Model file for the job. Use its own axes, mm. Round coordinates to 2 decimals unless told otherwise and drop trailing zeros. Order: outer loops, then holes, each group sorted by start corner. A loop starts at its lowest first (then second) coordinate and runs counter-clockwise, first axis right, second up. Notation, with made-up numbers: (9.25, 39.5) - (20.25, 39.5) arc R25 cw to (20.25, 76.5) - close; hole circle Ø1 at (-6.75, -3). An arc over 180 degrees is marked (long way). Put each result on its own line as item: value. Start each with the question number.
Item 1: Probe probe 1 along Z at (x, y) = (13.5, 3); probe 2 along Y at (x, z) = (36, 18). List the from-to ranges inside material, lowest first.
Item 2: Saw through at C-C on x = -21.5. List the corners of the cut face in (y, z).
Item 3: Saw through at A-A on y = 17.75. List the corners of the cut face in (x, z), plus the area to 3 significant figures.
Item 4: Pin check, flat tips, straight feed: pin 1 Ø10 at (x, y) = (-15.5, 17) entering from +Z; pin 2 Ø8 at (x, y) = (-10, 10.5) entering from +Z; pin 3 Ø4 at (y, z) = (4.5, -1) entering from +X; pin 4 Ø5 at (x, y) = (16.5, 7.5) entering from -Z. Stop position of each tip, or through.
Item 5: Saw through at B-B on z = -21.5. List the corners of the cut face in (x, y), plus the area to 3 significant figures.
```python
from build123d import *

# Parameters (mm, degrees)
SKETCH_1_W             = 100
SKETCH_1_H             = 100
EXTRUDE_1_DEPTH        = 1.5
SKETCH_2_R             = 0.75
EXTRUDE_2_DEPTH        = 0.75
SKETCH_3_W             = 1.5
SKETCH_3_H             = 3
EXTRUDE_3_DEPTH        = 1.5
SKETCH_5_W             = 3
SKETCH_5_H             = 1.5
EXTRUDE_4_DEPTH        = 3
SKETCH_7_R             = 0.75
EXTRUDE_5_DEPTH        = 2.5
SKETCH_8_W             = 6
SKETCH_8_H             = 9
EXTRUDE_6_DEPTH        = 10.4
SKETCH_9_W             = 3
SKETCH_9_H             = 1.5
EXTRUDE_7_DEPTH        = 4
SKETCH_10_R            = 0.75
EXTRUDE_8_DEPTH        = 3
SKETCH_11_W            = 6
SKETCH_11_H            = 2
CUT_EXTRUDE_1_DEPTH    = 10.4
SKETCH_12_W            = 6
SKETCH_12_H            = 3.5
EXTRUDE_9_DEPTH        = 20.17
SKETCH_13_W            = 3
SKETCH_13_H            = 1.5
EXTRUDE_10_DEPTH       = 4
SKETCH_14_R            = 0.75
EXTRUDE_11_DEPTH       = 2
PATTERN_LINEAR_2_COUNT = 2
PATTERN_LINEAR_2_PITCH = 13.6
SKETCH_16_W            = 6
SKETCH_16_H            = 8.75
CUT_EXTRUDE_2_DEPTH    = 9.25
SKETCH_17_W            = 6
SKETCH_17_H            = 2
CUT_EXTRUDE_3_DEPTH    = 1.65
SKETCH_18_W            = 3
SKETCH_18_H            = 1.5
EXTRUDE_12_DEPTH       = 4
SKETCH_19_R            = 0.75
EXTRUDE_13_DEPTH       = 3
EXTRUDE_14_DEPTH       = 1.5
SKETCH_21_W            = 0.75
SKETCH_21_H            = 3
CUT_EXTRUDE_4_DEPTH    = 1.5
SKETCH_22_W            = 1.5
SKETCH_22_H            = 0.5
EXTRUDE_15_DEPTH       = 2.5
SKETCH_23_W            = 3.5
SKETCH_23_H            = 14.4
CUT_EXTRUDE_5_DEPTH    = 6


with BuildPart() as part:
    # Sketch 1 → Extrude 1 (new body)
    with BuildSketch(Plane(origin=(0, 0, 0), x_dir=(1, 0, 0), z_dir=(0, 1, 0))):
        Rectangle(SKETCH_1_W, SKETCH_1_H)
    extrude(amount=EXTRUDE_1_DEPTH)



with BuildPart() as body_2:
    # Sketch 2 → Extrude 2 (new, symmetric)
    with BuildSketch(Plane.XY):
        with Locations((-40.336831864, 4.5)):
            Circle(SKETCH_2_R)
    extrude(amount=EXTRUDE_2_DEPTH, both=True)


with BuildPart() as part_1:
    add(part.part)

    add(body_2.part)  # Extrude 3 merges body 2
    # Sketch 3 → Extrude 3 (add)
    with BuildSketch(Plane.XY.offset(0.75)):
        with Locations((-40.336831864, 3)):
            Rectangle(SKETCH_3_W, SKETCH_3_H)
    extrude_3 = extrude(amount=EXTRUDE_3_DEPTH)

    # Mirror 1: Extrude 3 across plane
    add(extrude_3.mirror(Plane.XY))

    # Sketch 5 → Extrude 4 (add)
    with BuildSketch(Plane(origin=(0, 4.5, 0), x_dir=(1, 0, 0), z_dir=(0, 1, 0))):
        with Locations((-34.136831864, -0.5)):
            Rectangle(SKETCH_5_W, SKETCH_5_H)
        with Locations((-34.136831864, 3)):
            Rectangle(SKETCH_5_W, SKETCH_5_H)
    extrude(amount=-EXTRUDE_4_DEPTH)

    # Sketch 7 → Extrude 5 (add)
    with BuildSketch(Plane.XY.offset(-2.25)):
        with Locations(Location((-34.136831864, 4.5, 0), (0, 0, 180))):
            Circle(SKETCH_7_R)
    extrude(amount=EXTRUDE_5_DEPTH)

    # Sketch 8 → Extrude 6 (add)
    with BuildSketch(Plane(origin=(0, 1.5, 0), x_dir=(1, 0, 0), z_dir=(0, 1, 0))):
        with Locations((-17.336831864, 1.25)):
            Rectangle(SKETCH_8_W, SKETCH_8_H)
    extrude_6 = extrude(amount=EXTRUDE_6_DEPTH)

    # Sketch 9 → Extrude 7 (add)
    with BuildSketch(Plane(origin=(0, 11.9, 0), x_dir=(1, 0, 0), z_dir=(0, 1, 0))):
        with Locations((-17.336831864, 3)):
            Rectangle(SKETCH_9_W, SKETCH_9_H)
        with Locations((-17.336831864, -0.5)):
            Rectangle(SKETCH_9_W, SKETCH_9_H)
    extrude(amount=EXTRUDE_7_DEPTH)

    # Sketch 10 → Extrude 8 (add)
    with BuildSketch(Plane.XY.offset(-2.25)):
        with Locations(Location((-17.336831864, 14.9, 0), (0, 0, 180))):
            Circle(SKETCH_10_R)
    extrude(amount=EXTRUDE_8_DEPTH)

    # Sketch 11 → Cut-Extrude 1 (cut)
    with BuildSketch(Plane(origin=(0, 11.9, 0), x_dir=(1, 0, 0), z_dir=(0, 1, 0))):
        with Locations((-17.336831864, 1.25)):
            Rectangle(SKETCH_11_W, SKETCH_11_H)
    extrude(amount=-CUT_EXTRUDE_1_DEPTH, mode=Mode.SUBTRACT)

    # Sketch 12 → Extrude 9 (add)
    with BuildSketch(Plane(origin=(0, 1.5, 0), x_dir=(1, 0, 0), z_dir=(0, 1, 0))):
        with Locations((16.243168136, 0)):
            Rectangle(SKETCH_12_W, SKETCH_12_H)
        with Locations((16.243168136, 5.5)):
            Rectangle(SKETCH_12_W, SKETCH_12_H)
    extrude(amount=EXTRUDE_9_DEPTH)

    # Sketch 13 → Extrude 10 (add)
    with BuildSketch(Plane(origin=(0, 21.67, 0), x_dir=(1, 0, 0), z_dir=(0, 1, 0))):
        with Locations((16.243168136, 1)):
            Rectangle(SKETCH_13_W, SKETCH_13_H)
        with Locations((16.243168136, 4.5)):
            Rectangle(SKETCH_13_W, SKETCH_13_H)
    extrude(amount=EXTRUDE_10_DEPTH)

    # Sketch 14 → Extrude 11 (add)
    with BuildSketch(Plane.XY.offset(-3.75)):
        with Locations(Location((16.243168136, 24.67, 0), (0, 0, 180))):
            Circle(SKETCH_14_R)
    extrude(amount=EXTRUDE_11_DEPTH)

    # Pattern Linear 2: Extrude 6 ×2
    with Locations(*[(i * PATTERN_LINEAR_2_PITCH, 0, 0) for i in range(1, PATTERN_LINEAR_2_COUNT)]):
        add(extrude_6)

    # Sketch 16 → Cut-Extrude 2 (cut, symmetric)
    with BuildSketch(Plane.XY):
        with Locations((-3.736831864, 7.525)):
            Rectangle(SKETCH_16_W, SKETCH_16_H)
    extrude(amount=CUT_EXTRUDE_2_DEPTH, both=True, mode=Mode.SUBTRACT)

    # Sketch 17 → Cut-Extrude 3 (cut)
    with BuildSketch(Plane(origin=(0, 3.15, 0), x_dir=(1, 0, 0), z_dir=(0, 1, 0))):
        with Locations((-3.736831864, 1.25)):
            Rectangle(SKETCH_17_W, SKETCH_17_H)
    extrude(amount=-CUT_EXTRUDE_3_DEPTH, mode=Mode.SUBTRACT)

    # Sketch 18 → Extrude 12 (add)
    with BuildSketch(Plane(origin=(0, 3.15, 0), x_dir=(1, 0, 0), z_dir=(0, 1, 0))):
        with Locations((-3.736831864, 3)):
            Rectangle(SKETCH_18_W, SKETCH_18_H)
        with Locations((-3.736831864, -0.5)):
            Rectangle(SKETCH_18_W, SKETCH_18_H)
    extrude(amount=EXTRUDE_12_DEPTH)

    # Sketch 19 → Extrude 13 (add)
    with BuildSketch(Plane.XY.offset(-2.25)):
        with Locations(Location((-3.736831864, 6.15, 0), (0, 0, 180))):
            Circle(SKETCH_19_R)
    extrude(amount=EXTRUDE_13_DEPTH)

    # Sketch 20 → Extrude 14 (add)
    with BuildSketch(Plane(origin=(0, 4.5, 0), x_dir=(1, 0, 0), z_dir=(0, 1, 0))):
        Polygon((-32.636831864, 0.25), (-33.386831864, 0.25), (-33.386831864, -0.25), (-34.886831864, -0.25), (-34.886831864, 0.25), (-35.636831864, 0.25), (-35.636831864, -1.25), (-32.636831864, -1.25), align=None)
        Polygon((-35.636831864, 3.75), (-35.636831864, 2.25), (-34.886831864, 2.25), (-33.386831864, 2.25), (-32.636831864, 2.25), (-32.636831864, 3.75), align=None)
    extrude(amount=EXTRUDE_14_DEPTH)

    # Sketch 21 → Cut-Extrude 4 (cut)
    with BuildSketch(Plane.ZY.offset(41.086831864)):
        with Locations((1.875, 3)):
            Rectangle(SKETCH_21_W, SKETCH_21_H)
        with Locations((-1.875, 3)):
            Rectangle(SKETCH_21_W, SKETCH_21_H)
    extrude(amount=-CUT_EXTRUDE_4_DEPTH, mode=Mode.SUBTRACT)

    # Sketch 22 → Extrude 15 (add)
    with BuildSketch(Plane(origin=(0, 6, 0), x_dir=(1, 0, 0), z_dir=(0, 1, 0))):
        with Locations((-34.136831864, 0)):
            Rectangle(SKETCH_22_W, SKETCH_22_H)
    extrude(amount=-EXTRUDE_15_DEPTH)

    # Sketch 23 → Cut-Extrude 5 (cut)
    with BuildSketch(Plane.ZY.offset(20.336831864)):
        with Locations((-4, 8.7)):
            Rectangle(SKETCH_23_W, SKETCH_23_H)
    extrude(amount=-CUT_EXTRUDE_5_DEPTH, mode=Mode.SUBTRACT)


solid = part_1.part
```
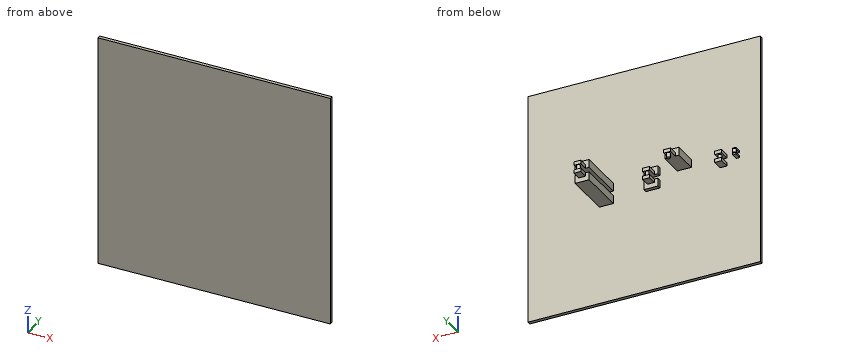
Results found:
1. probe 1: z = -7.25 to -3.75, -1.75 to 1.75
1. probe 2: y = 0 to 1.5
2. outline: (0, -50) - (1.5, -50) - (1.5, 50) - (0, 50) - close
3. outline: (13.24, -7.25) - (19.24, -7.25) - (19.24, -3.75) - (13.24, -3.75) - close; (13.24, -1.75) - (19.24, -1.75) - (19.24, 1.75) - (13.24, 1.75) - close
3. area: 42.0 mm²
4. pin 1: stops at z = 1.25
4. pin 2: passes through
4. pin 3: stops at x = 19.24
4. pin 4: stops at z = -7.25
5. outline: (-50, 0) - (50, 0) - (50, 1.5) - (-50, 1.5) - close
5. area: 150 mm²
